from build123d import *

# Parameters (mm, degrees)
BOSS_EXTRUDE2_DEPTH            = 7
BOSS_EXTRUDE3_DEPTH            = 2
CUT_EXTRUDE1_DEPTH             = 1.25
SKETCH6_R                      = 2.5
BOSS_EXTRUDE4_DEPTH            = 2
BOSS_EXTRUDE5_DEPTH            = 1.5
SKETCH7_R                      = 2.5
CUT_EXTRUDE2_DEPTH             = 19.823190484
SKETCH18_R                     = 0.625
CUT_EXTRUDE5_DEPTH             = 8.5
CUT_EXTRUDE6_REACH             = 24.439
SKETCH20_R                     = 0.625
CUT_EXTRUDE6_DIRECTION_2_REACH = 24.439


with BuildPart() as part:
    # Sketch3 → Boss-Extrude2 (new body)
    with BuildSketch(Plane(origin=(0, 0, 0), x_dir=(1, 0, 0), z_dir=(0, 1, 0))):
        with BuildLine():
            Line((-6, -8), (6, -8))
            ThreePointArc((6, -8), (7.414213562, -7.414213562), (8, -6))
            Line((8, -6), (8, 6))
            ThreePointArc((8, 6), (7.414213562, 7.414213562), (6, 8))
            Line((6, 8), (-6, 8))
            ThreePointArc((-6, 8), (-7.414213562, 7.414213562), (-8, 6))
            Line((-8, 6), (-8, -6))
            ThreePointArc((-8, -6), (-7.414213562, -7.414213562), (-6, -8))
        make_face()
    extrude(amount=BOSS_EXTRUDE2_DEPTH)

    # Sketch4 → Boss-Extrude3 (add)
    with BuildSketch(Plane(origin=(0, 7, 0), x_dir=(1, 0, 0), z_dir=(0, 1, 0))):
        with BuildLine():
            Line((-15.5, 0), (-8, 0))
            Line((-8, 0), (-8, 3.465))
            Line((-8, 3.465), (-15, 3.465))
            ThreePointArc((-15, 3.465), (-15.353553391, 3.318553391), (-15.5, 2.965))
            Line((-15.5, 2.965), (-15.5, 0))
        make_face()
        with BuildLine():
            Line((-8, -3.465), (-8, 0))
            Line((-8, 0), (-15.5, 0))
            Line((-15.5, 0), (-15.5, -2.965))
            ThreePointArc((-15.5, -2.965), (-15.353553391, -3.318553391), (-15, -3.465))
            Line((-15, -3.465), (-8, -3.465))
        make_face()
        with BuildLine():
            Line((15, 3.465), (8, 3.465))
            Line((8, 3.465), (8, 0))
            Line((8, 0), (15.5, 0))
            Line((15.5, 0), (15.5, 2.965))
            ThreePointArc((15.5, 2.965), (15.353553391, 3.318553391), (15, 3.465))
        make_face()
        with BuildLine():
            Line((15.5, 0), (8, 0))
            Line((8, 0), (8, -3.465))
            Line((8, -3.465), (15, -3.465))
            ThreePointArc((15, -3.465), (15.353553391, -3.318553391), (15.5, -2.965))
            Line((15.5, -2.965), (15.5, 0))
        make_face()
    extrude(amount=-BOSS_EXTRUDE3_DEPTH)

    # Sketch5 → Cut-Extrude1 (cut)
    with BuildSketch(Plane(origin=(0, 7, 0), x_dir=(1, 0, 0), z_dir=(0, 1, 0))):
        with BuildLine():
            Line((-3.5, 2.5), (-14.25, 2.5))
            ThreePointArc((-14.25, 2.5), (-14.603553391, 2.353553391), (-14.75, 2))
            Line((-14.75, 2), (-14.75, -2))
            ThreePointArc((-14.75, -2), (-14.603553391, -2.353553391), (-14.25, -2.5))
            Line((-14.25, -2.5), (-3.5, -2.5))
            ThreePointArc((-3.5, -2.5), (-1, 0), (-3.5, 2.5))
        make_face()
        with BuildLine():
            Line((3.5, 2.5), (14.25, 2.5))
            ThreePointArc((14.25, 2.5), (14.603553391, 2.353553391), (14.75, 2))
            Line((14.75, 2), (14.75, -2))
            ThreePointArc((14.75, -2), (14.603553391, -2.353553391), (14.25, -2.5))
            Line((14.25, -2.5), (3.5, -2.5))
            ThreePointArc((3.5, -2.5), (1, 0), (3.5, 2.5))
        make_face()
    extrude(amount=-CUT_EXTRUDE1_DEPTH, mode=Mode.SUBTRACT)

    # Sketch6 → Boss-Extrude4 (add)
    with BuildSketch(Plane(origin=(0, 7, 0), x_dir=(1, 0, 0), z_dir=(0, 1, 0))):
        with BuildLine():
            Line((-6, -8), (6, -8))
            ThreePointArc((6, -8), (7.414213562, -7.414213562), (8, -6))
            Line((8, -6), (8, 6))
            ThreePointArc((8, 6), (7.414213562, 7.414213562), (6, 8))
            Line((6, 8), (-6, 8))
            ThreePointArc((-6, 8), (-7.414213562, 7.414213562), (-8, 6))
            Line((-8, 6), (-8, -6))
            ThreePointArc((-8, -6), (-7.414213562, -7.414213562), (-6, -8))
        make_face()
        with Locations(Location((3.5, 0, 0), (0, 0, 270))):
            Circle(SKETCH6_R, mode=Mode.SUBTRACT)
        with Locations(Location((-3.5, 0, 0), (0, 0, 270))):
            Circle(SKETCH6_R, mode=Mode.SUBTRACT)
    extrude(amount=BOSS_EXTRUDE4_DEPTH)

    # Sketch8 → Boss-Extrude5 (add)
    with BuildSketch(Plane.XZ):
        with BuildLine():
            Line((-7, -9), (7, -9))
            ThreePointArc((7, -9), (8.414213562, -8.414213562), (9, -7))
            Line((9, -7), (9, 7))
            ThreePointArc((9, 7), (8.414213562, 8.414213562), (7, 9))
            Line((7, 9), (-7, 9))
            ThreePointArc((-7, 9), (-8.414213562, 8.414213562), (-9, 7))
            Line((-9, 7), (-9, -7))
            ThreePointArc((-9, -7), (-8.414213562, -8.414213562), (-7, -9))
        make_face()
    extrude(amount=-BOSS_EXTRUDE5_DEPTH)

    # Sketch7 → Cut-Extrude2 (cut, through all)
    with BuildSketch(Plane(origin=(0, 5.75, 0), x_dir=(1, 0, 0), z_dir=(0, 1, 0))):
        with Locations(Location((-3.5, 0, 0), (0, 0, 270))):
            Circle(SKETCH7_R)
        with Locations(Location((3.5, 0, 0), (0, 0, 270))):
            Circle(SKETCH7_R)
    extrude(amount=-CUT_EXTRUDE2_DEPTH, mode=Mode.SUBTRACT)

    # Sketch13 → Revolve1 (revolve)
    with BuildSketch(Plane(origin=(0, 0, 0), x_dir=(0, 0, -1), z_dir=(1, 0, 0)), mode=Mode.PRIVATE) as revolve1_sk:
        Polygon((-8, 3.479112133), (-13.5, 3.479112133), (-13.5, 2.979112133), (-11, 2.525029687), (-11, 2.879112133), (-8, 2.879112133), align=None)
    revolve(revolve1_sk.sketch.rotate(Axis((0, 4.104112133, 8), (0, 0, 1)), 180), axis=Axis((0, 4.104112133, 8), (0, 0, 1)))

    # Sketch18 → Cut-Extrude5 (cut)
    with BuildSketch(Plane.XY.offset(8)):
        with Locations(Location((0, 4.104112133, 0), (0, 0, 90))):
            Circle(SKETCH18_R)
    extrude(amount=-CUT_EXTRUDE5_DEPTH, mode=Mode.SUBTRACT)

    # Sketch20 → Cut-Extrude6 (cut, up to next)
    with BuildSketch(Plane(origin=(0, 0, 0), x_dir=(0, 0, -1), z_dir=(1, 0, 0)), mode=Mode.PRIVATE) as cut_extrude6_sk1:
        with Locations(Location((0.5, 4.104112133, 0), (0, 0, 180))):
            Circle(SKETCH20_R)
    cut_extrude6_tool1 = extrude(cut_extrude6_sk1.sketch, amount=-CUT_EXTRUDE6_REACH, mode=Mode.PRIVATE) & part.part
    add(cut_extrude6_tool1.solids().sort_by_distance((0, 4.104112, -0.5))[0], mode=Mode.SUBTRACT)

    # Sketch20 → Cut-Extrude6 direction 2 (cut, up to next)
    with BuildSketch(Plane(origin=(0, 0, 0), x_dir=(0, 0, -1), z_dir=(1, 0, 0)), mode=Mode.PRIVATE) as cut_extrude6_direction_2_sk1:
        with Locations(Location((0.5, 4.104112133, 0), (0, 0, 180))):
            Circle(SKETCH20_R)
    cut_extrude6_direction_2_tool1 = extrude(cut_extrude6_direction_2_sk1.sketch, amount=CUT_EXTRUDE6_DIRECTION_2_REACH, mode=Mode.PRIVATE) & part.part
    add(cut_extrude6_direction_2_tool1.solids().sort_by_distance((0, 4.104112, -0.5))[0], mode=Mode.SUBTRACT)


solid = part.part
CAD build for the part. Positions are in the model's coordinates, mm. A direction names the side the tool comes from. Round coordinates to 2 decimals unless told otherwise and drop trailing zeros. Write each loop counter-clockwise with the first axis right and the second up, starting at its lowest first coordinate (ties: lowest second). Pieces come first, ordered by that corner, then holes.
(1) Slice it at C-C, the plane x = -13. Write the cut outline in (y, z) (3 decimals).
(2) Slice it at B-B, the plane y = 0.75. Write the cut outline in (x, z), and give its area (3 significant figures).
(3) Slice it at A-A, the plane x = 2. Write the cut outline in (y, z).
(4) 3-axis set-ups, long thin cutter, end or side, ignore diameter. For faces 5 (the face through (0, 5, -8)), 6 (the face through (7.4, 5.2, 7.43)), 7 (the face through (-9, 6, 2.5)): which of +Z, -Z, +X, -X, +Y, -Y reach the whole face in a straight line?
(5) Probe line 1 along Z through (x, y) = (-5, 4.75); line 2 along Y through (x, z) = (-0.65, -0.5); line 3 along Z through (x, y) = (-3.5, 4.5). List the from-to ranges inside material, lowest first.
(6) Slice it at D-D, the plane z = -7.5. Write the cut outline in (x, y).
(7) Drop flat-ended pins along their axis: P1, Ø5, axis at y = 4.5, z = -5.5, coming from the -X side; P2, Ø1.6, axis at x = 12.5, y = 6.5, coming from the +Z side (3 decimals); P3, Ø2.5, axis at x = -1, y = 3.5, coming from the -Z side; P4, Ø3, axis at x = 11.5, y = 3, coming from the -Z side. Give the stop position or say it passes through.
(8) Mould opens along Z. For faces 1 (the face through (0, 9, 0)), 2 (the face through (0, 5, 13.5)), 3 (the face through (12, 6, -3.465)), 4 (the face through (10, 5.75, 0)) say: pulls with the +Z half, pulls with the -Z half, needs draft (parallel to the pull), parting line crosses it, or undercut.
From the geometry:
1. outline: (5, -3.465) - (7, -3.465) - (7, -2.5) - (5.75, -2.5) - (5.75, 2.5) - (7, 2.5) - (7, 3.465) - (5, 3.465) - close
2. outline: (-9, -7) arc R2 ccw to (-7, -9) - (7, -9) arc R2 ccw to (9, -7) - (9, 7) arc R2 ccw to (7, 9) - (-7, 9) arc R2 ccw to (-9, 7) - close; hole circle Ø5 at (-3.5, 0); hole circle Ø5 at (3.5, 0)
2. area: 281 mm2
3. outline: (0, -9) - (1.5, -9) - (1.5, -8) - (9, -8) - (9, -2) - (0, -2) - close; (0, 2) - (9, 2) - (9, 8) - (1.5, 8) - (1.5, 9) - (0, 9) - close
4. face 5: -Z, +X, -X, +Y
4. face 6: +Z, +X, +Y
4. face 7: none
5. line 1: z = -8 to -2, 2 to 8
5. line 2: y = 0 to 3.48, 4.73 to 9
5. line 3: z = -8 to -2.5, 2.5 to 8
6. outline: (-8.94, 0) - (8.94, 0) - (8.94, 1.5) - (7.32, 1.5) - (7.32, 9) - (-7.32, 9) - (-7.32, 1.5) - (-8.94, 1.5) - close
7. P1: stops at x = -15.49
7. P2: stops at z = 3.465
7. P3: stops at z = -8
7. P4: passes through
8. face 1: needs draft
8. face 2: pulls with the +Z half
8. face 3: pulls with the -Z half
8. face 4: undercut
